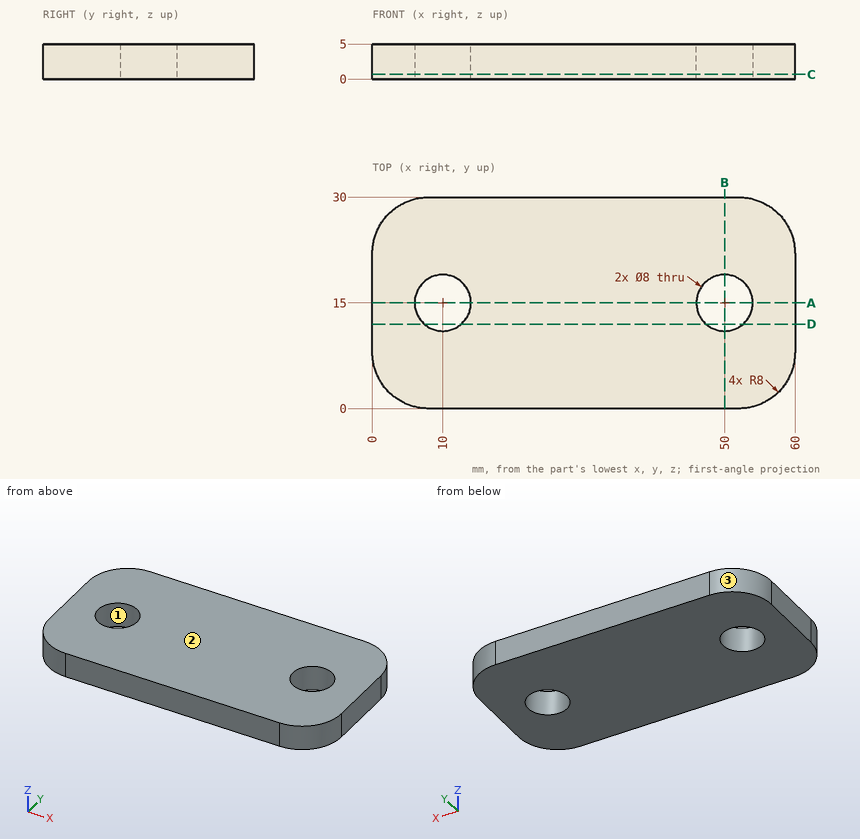
Here's the drawing with two shaded views (mm, measured from the low corner). I have some questions. Give positions to 0.01 mm unless a question says otherwise; leave off trailing zeros. Loops run counter-clockwise (first coordinate to the right, second up) from the corner with the lowest first, then second, coordinate; pieces in that order, holes last. Notation, with made-up numbers: M -28.75,84.5 L 8.25,84.5 A24 cw 8.25,109.5 Z; hole C 44,14 d2. An arc over 180 degrees is marked long. Use one line per item in the form item = value. Start each with the question number.
Q1. Thinking about a two-plate mould opening in Y: for the marked faces 1, 2 and 3, which applies, +Y half, -Y half, draft (parallel to the pull), parting line (faces both ways), or undercut?
Q2. If we section it at B-B (x = 50): Write out the boundary of the cut face in (y, z).
Q3. If we section it at C-C (z = 0.7): Write out the boundary of the cut face in (x, y), then the cut area to 3 significant figures.
Q4. If we section it at A-A (y = 15): Write out the boundary of the cut face in (x, z), then the cut area to 3 significant figures.
Q5. I need wall thicknesses on line 1 along X through (y, z) = (15.25, 3.25); line 2 along Y through (x, z) = (50, 1.25); line 3 along Y through (x, z) = (8, 4). Which ranges of each line are inside material? Lowest first, please.
Q6. If we section it at D-D (y = 12): Write out the boundary of the cut face in (x, z).
Q7. Will this pin go through, and if not, where does the flat tip stop? pin 1 Ø10.5 at (x, y) = (50, 15) entering from -Z.
Taken from the geometry:
q1.face_1 = undercut
q1.face_2 = draft
q1.face_3 = +Y half
q2.outline = M 0,0 L 11,0 L 11,5 L 0,5 Z; M 19,0 L 30,0 L 30,5 L 19,5 Z
q3.outline = M 0,8 A8 ccw 8,0 L 52,0 A8 ccw 60,8 L 60,22 A8 ccw 52,30 L 8,30 A8 ccw 0,22 Z; hole C 10,15 d8; hole C 50,15 d8
q3.area = 1,640 mm^2
q4.outline = M 0,0 L 6,0 L 6,5 L 0,5 Z; M 14,0 L 46,0 L 46,5 L 14,5 Z; M 54,0 L 60,0 L 60,5 L 54,5 Z
q4.area = 220 mm^2
q5.line_1 = 0 to 6.01, 13.99 to 46.01, 53.99 to 60
q5.line_2 = 0 to 11, 19 to 30
q5.line_3 = 0 to 11.54, 18.46 to 30
q6.outline = M 0,0 L 7.35,0 L 7.35,5 L 0,5 Z; M 12.65,0 L 47.35,0 L 47.35,5 L 12.65,5 Z; M 52.65,0 L 60,0 L 60,5 L 52.65,5 Z
q7.pin_1 = 0
